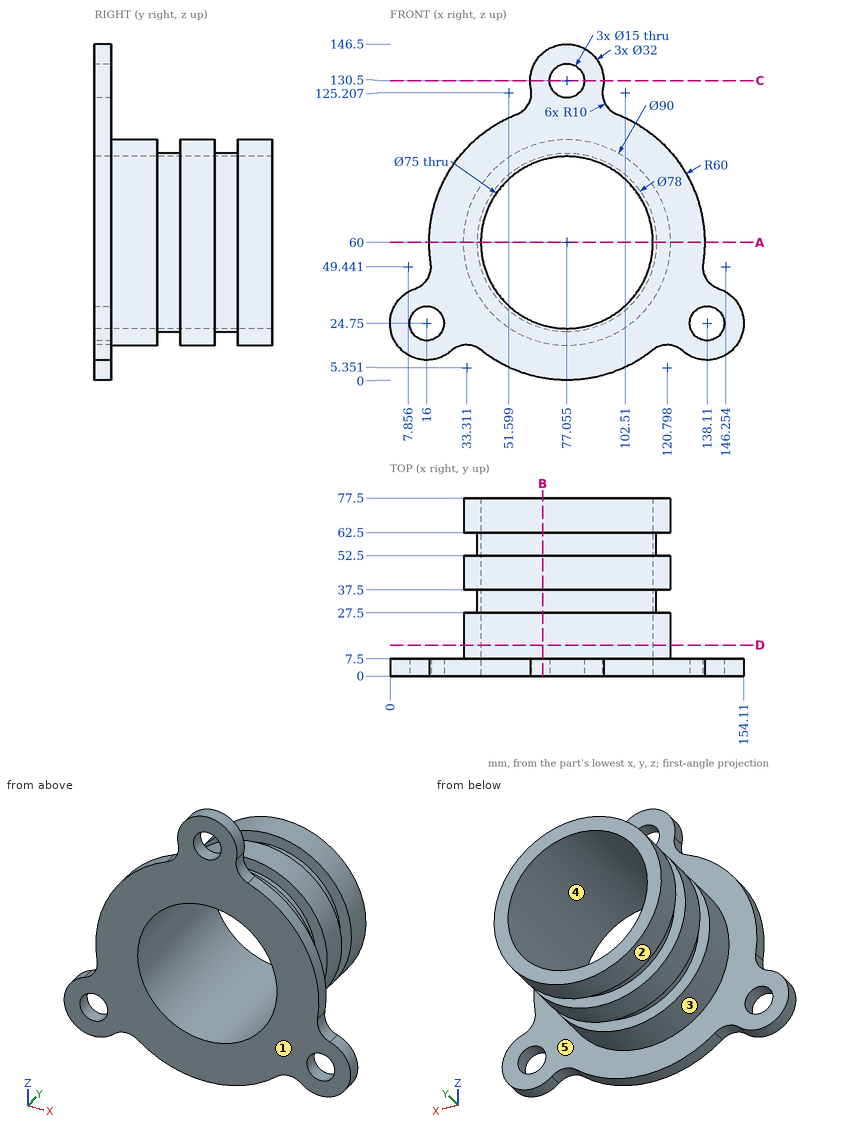
Part print with two shaded views. Sizes in mm from the minimum x, y, z corner. A direction names the side the tool comes from. Round coordinates to 2 decimals unless told otherwise and drop trailing zeros. Loops run counter-clockwise (first coordinate to the right, second up) from the corner with the lowest first, then second, coordinate; pieces in that order, holes last. Notation, with made-up numbers: M -34.5,2 L 21.5,2 A29 cw 21.5,29 Z; hole C -23,-24.75 d10. An arc over 180 degrees is marked long. Return JSON: item names as keys, results as strings. Group by question number.
(1) Mould opens along Z. For the marked faces 3, 4 and 5 say: +Z half, -Z half, draft (parallel to the pull), parting line (faces both ways), or undercut.
(2) Saw through at B-B, the plane x = 66.5. List the corners of the cut face in (y, z) (1 decimal).
(3) Drop flat-ended pins along their axis: P1, Ø4, axis at y = 33, z = 80, coming from the -X side; P2, Ø12, axis at x = 113, y = 12, coming from the +Z side; P3, Ø12, axis at x = 31.5, y = 26.5, coming from the -Z side (1 decimal). Give the stop position or say it passes through.
(4) Saw through at C-C, the plane z = 130.5. List the corners of the cut face in (x, y) (1 decimal).
(5) Saw through at A-A, the plane z = 60. List the corners of the cut face in (x, y) (1 decimal), and give its area (3 significant figures).
(6) Wall check: probe 1 along Y at (x, z) = (110, 33); probe 2 along X at (y, z) = (3.25, 130.5) (1 decimal); probe 3 along Y at (x, z) = (100, 15.5). Give the ranges that are in metal, low to high. Write a range as [from, to].
(7) Saw through at D-D, the plane y = 13.5. List the corners of the cut face in (x, z) (1 decimal), and give its area (3 significant figures).
(8) Tool access for the marked faces 1 and 2: list every direction of +Z, -Z, +X, -X, +Y, -Y with a clear straight run to the whole face (end or side of a thin tool).
Answer list:
{
 "1": {"face 3": "parting line", "face 4": "undercut", "face 5": "draft"},
 "2": {"outline": "M 0,0.9 L 7.5,0.9 L 7.5,16.3 L 27.5,16.3 L 27.5,22.5 L 37.5,22.5 L 37.5,16.3 L 52.5,16.3 L 52.5,22.5 L 62.5,22.5 L 62.5,16.3 L 77.5,16.3 L 77.5,24 L 0,24 Z; M 0,96 L 77.5,96 L 77.5,103.7 L 62.5,103.7 L 62.5,97.5 L 52.5,97.5 L 52.5,103.7 L 37.5,103.7 L 37.5,97.5 L 27.5,97.5 L 27.5,103.7 L 7.5,103.7 L 7.5,142.5 L 0,142.5 Z"},
 "3": {"P1": "x = 42.46", "P2": "z = 110.77", "P3": "z = 38.5"},
 "4": {"outline": "M 61.1,0 L 69.6,0 L 69.6,7.5 L 61.1,7.5 Z; M 84.6,0 L 93.1,0 L 93.1,7.5 L 84.6,7.5 Z"},
 "5": {"outline": "M 17.1,0 L 39.6,0 L 39.6,77.5 L 32.1,77.5 L 32.1,62.5 L 38.1,62.5 L 38.1,52.5 L 32.1,52.5 L 32.1,37.5 L 38.1,37.5 L 38.1,27.5 L 32.1,27.5 L 32.1,7.5 L 17.1,7.5 Z; M 114.6,0 L 137.1,0 L 137.1,7.5 L 122.1,7.5 L 122.1,27.5 L 116.1,27.5 L 116.1,37.5 L 122.1,37.5 L 122.1,52.5 L 116.1,52.5 L 116.1,62.5 L 122.1,62.5 L 122.1,77.5 L 114.6,77.5 Z", "area": "1,150 mm2"},
 "6": {"probe 1": "[0, 27.5], [37.5, 52.5], [62.5, 77.5]", "probe 2": "[61.1, 69.6], [84.6, 93.1]", "probe 3": "[0, 7.5]"},
 "7": {"outline": "C 77.1,60 d90; hole C 77.1,60 d75", "area": "1,940 mm2"},
 "8": {"face 1": "+Z, -Z, +X, -X, -Y", "face 2": "+Y"}
}
